Could you check a few things on this model? Use its own coordinates, in mm. A direction names the side the tool comes from. Give positions to 0.01 mm unless a question says otherwise; leave off trailing zeros. Order: outer loops, then holes, each group sorted by start corner. A loop starts at its lowest first (then second) coordinate and runs counter-clockwise, first axis right, second up.
(1) If we mould it in two halves opening along Y, with no side actions, what happens to faces 1 (the flat face through (-15, -9.35, 59)), 2 (the flat face through (42.605, 0.49, 34.51))? For each: released by +Y, released by -Y, zero draft, split by the parting line, or undercut.
(2) Imagine slicing it at B-B, the plane x = 0. Write out the boundary of the cut face in (y, z), then the cut area to 3 significant figures.
(3) Will these pins go through, and if not, where does the flat tip stop? pin 1 (10 mm diameter, centred on x = -3.5, y = 6.5, fed in from -Z); pin 2 (3.5 mm diameter, centred on y = 33, z = 7.5, fed in from +X); pin 3 (4 mm diameter, centred on y = -22, z = 12.5, fed in from +X).
(4) Imagine slicing it at A-A, the plane y = 0. Write out the boundary of the cut face in (x, z), then the cut area to 3 significant figures.
(5) If I drill on probe 1 along Y at (x, z) = (-17.5, 52.6); probe 2 along X at (y, z) = (14.5, 52); probe 3 along Y at (x, z) = (-18, 65), over which ranges is the centre line in solid material (lowest first)?
(6) Imagine slicing it at D-D, the plane x = -17.5. Write out the boundary of the cut face in (y, z), then the cut area to 3 significant figures.
(7) On a 3-axis mill with a long thin cutter (end or side, diameter ignored), from which of +Z, -Z, +X, -X, +Y, -Y can I reach the whole of each face in a straight line? I mean faces 3 (the flat face through (-33, 0, 3)), 4 (the flat face through (21, 7, 55)), 5 (the flat face through (18, 8, 54.7)), 6 (the flat face through (32, 34, 8)). Say none if no direction works.
(8) Imagine slicing it at C-C, the plane z = 17. Write out the boundary of the cut face in (x, y), then the cut area to 3 significant figures.
from build123d import *

# Parameters (mm, degrees)
SCHIZZO1_W                   = 70
SCHIZZO1_H                   = 70
ESTRUSIONE_ESTRUSIONE1_DEPTH = 70
SCHIZZO3_W                   = 64
SCHIZZO3_H                   = 64
TAGLIO_ESTRUSIONE2_DEPTH     = 67
TAGLIO_ESTRUSIONE1_REACH     = 87.732
SCHIZZO2_R                   = 3.65
TAGLIO_ESTRUSIONE3_START     = -70
SCHIZZO4_W                   = 64
SCHIZZO4_H                   = 64
TAGLIO_ESTRUSIONE3_DEPTH     = 70
SPECCHIA2_START              = -70
SPECCHIA2_COPY_1_SKETCH_W    = 64
SPECCHIA2_COPY_1_SKETCH_H    = 64
SPECCHIA2_COPY_1_DEPTH       = 70
ESTRUSIONE_ESTRUSIONE2_DEPTH = 15.3
SCHIZZO6_R                   = 1.5
TAGLIO_ESTRUSIONE4_DEPTH     = 3
SCHIZZO7_W                   = 42
SCHIZZO7_H                   = 14
SCHIZZO7_H_2                 = 11.35
ESTRUSIONE_ESTRUSIONE3_DEPTH = 8
SCHIZZO8_W                   = 15
SCHIZZO8_H                   = 70


with BuildPart() as part:
    # Schizzo1 → Estrusione-Estrusione1 (new body)
    with BuildSketch(Plane.XY):
        Rectangle(SCHIZZO1_W, SCHIZZO1_H)
    extrude(amount=ESTRUSIONE_ESTRUSIONE1_DEPTH)

    # Schizzo3 → Taglio-Estrusione2 (cut)
    with BuildSketch(Plane(origin=(0, 0, 0), x_dir=(-1, 0, 0), z_dir=(0, 0, -1))):
        Rectangle(SCHIZZO3_W, SCHIZZO3_H)
    extrude(amount=-TAGLIO_ESTRUSIONE2_DEPTH, mode=Mode.SUBTRACT)

    # Schizzo2 → Taglio-Estrusione1 (cut, up to next)
    with BuildSketch(Plane.XY.offset(70), mode=Mode.PRIVATE) as taglio_estrusione1_sk1:
        Circle(SCHIZZO2_R)
    taglio_estrusione1_tool1 = extrude(taglio_estrusione1_sk1.sketch, amount=-TAGLIO_ESTRUSIONE1_REACH, mode=Mode.PRIVATE) & part.part
    add(taglio_estrusione1_tool1.solids().sort_by_distance((0, 0, 70))[0], mode=Mode.SUBTRACT)

    # Schizzo4 → Taglio-Estrusione3 (cut)
    with BuildSketch(Plane.XZ.offset(35).offset(TAGLIO_ESTRUSIONE3_START)):
        with Locations((0, 35)):
            Rectangle(SCHIZZO4_W, SCHIZZO4_H)
    taglio_estrusione3 = extrude(amount=TAGLIO_ESTRUSIONE3_DEPTH, mode=Mode.SUBTRACT)

    # Specchia1: Taglio-Estrusione3 across plane
    add(taglio_estrusione3.mirror(Plane(origin=(0, 0, 0), x_dir=(0, 0, 1), z_dir=(-0.7071067811865476, 0.7071067811865475, 0))), mode=Mode.SUBTRACT)

    # Specchia2: Taglio-Estrusione3 across plane
    add(taglio_estrusione3.mirror(Plane(origin=(0, 0, 0), x_dir=(0, 0, 1), z_dir=(-0.7071067811865476, 0.7071067811865475, 0))), mode=Mode.SUBTRACT)

    # Specchia2 copy 1 sketch → Specchia2 copy 1 (cut)
    with BuildSketch(Plane.XZ.offset(35).offset(SPECCHIA2_START)):
        with Locations((0, 35)):
            Rectangle(SPECCHIA2_COPY_1_SKETCH_W, SPECCHIA2_COPY_1_SKETCH_H)
    extrude(amount=SPECCHIA2_COPY_1_DEPTH, mode=Mode.SUBTRACT)

    # Schizzo5 → Estrusione-Estrusione2 (add)
    with BuildSketch(Plane(origin=(0, 0, 67), x_dir=(-1, 0, 0), z_dir=(0, 0, -1))):
        Polygon((-21, 23.65), (21, 23.65), (21, -9.35), (8, -9.35), (8, 4.65), (-8, 4.65), (-8, -9.35), (-21, -9.35), align=None)
    extrude(amount=ESTRUSIONE_ESTRUSIONE2_DEPTH)

    # Schizzo6 → Taglio-Estrusione4 (cut)
    with BuildSketch(Plane(origin=(0, 0, 51.7), x_dir=(-1, 0, 0), z_dir=(0, 0, -1))):
        with Locations((-17.5, 7.5)):
            Circle(SCHIZZO6_R)
        with Locations(Location((17.5, 7.5, 0), (0, 0, 180))):
            Circle(SCHIZZO6_R)
    extrude(amount=-TAGLIO_ESTRUSIONE4_DEPTH, mode=Mode.SUBTRACT)

    # Schizzo7 → Estrusione-Estrusione3 (add)
    with BuildSketch(Plane(origin=(0, 0, 67), x_dir=(-1, 0, 0), z_dir=(0, 0, -1))):
        with Locations((0, -28)):
            Rectangle(SCHIZZO7_W, SCHIZZO7_H)
        Polygon((32, 32), (32, 35), (21, 35), (21, 23.65), (21, -9.35), (21, -21), (21, -35), (32, -35), (32, -32), (35, -32), (35, 32), align=None)
        with Locations((0, 29.325)):
            Rectangle(SCHIZZO7_W, SCHIZZO7_H_2)
        Polygon((-21, 23.65), (-21, 35), (-32, 35), (-32, 32), (-35, 32), (-35, -32), (-32, -32), (-32, -35), (-21, -35), (-21, -21), (-21, -9.35), align=None)
    extrude(amount=ESTRUSIONE_ESTRUSIONE3_DEPTH)

    # Sweep1: sweep along a path in Schizzo9
    with BuildLine(Plane.XZ.offset(35)) as sweep1_path:
        Line((35, 70), (50, 0))
    # Schizzo8 → Sweep1 (sweep)
    with BuildSketch(Plane(origin=(0, 0, 0), x_dir=(-1, 0, 0), z_dir=(0, 0, -1))):
        with Locations((-42.5, 0)):
            Rectangle(SCHIZZO8_W, SCHIZZO8_H)
    sweep1 = sweep(path=sweep1_path.line)

    # Specchia4: Sweep1 across plane
    add(sweep1.mirror(Plane(origin=(0, 0, 0), x_dir=(0, 0, 1), z_dir=(1, 0, 0))))


solid = part.part
Answer block:
1. face 1: undercut
1. face 2: zero draft
2. outline: (-35, 0) - (-32, 0) - (-32, 3) - (-35, 3) - close; (-35, 59) - (-21, 59) - (-21, 67) - (-3.65, 67) - (-3.65, 70) - (-35, 70) - close; (3.65, 67) - (4.65, 67) - (4.65, 51.7) - (23.65, 51.7) - (23.65, 59) - (35, 59) - (35, 70) - (3.65, 70) - close; (32, 0) - (35, 0) - (35, 3) - (32, 3) - close
2. area: 700 mm2
3. pin 1: stops at z = 51.7
3. pin 2: stops at x = 48.77
3. pin 3: stops at x = 47.75
4. outline: (-50, 0) - (-32, 0) - (-32, 3) - (-34.36, 3) - (-22.36, 59) - (-21, 59) - (-21, 51.7) - (-8, 51.7) - (-8, 67) - (-3.65, 67) - (-3.65, 70) - (-35, 70) - close; (3.65, 67) - (8, 67) - (8, 51.7) - (21, 51.7) - (21, 59) - (22.36, 59) - (34.36, 3) - (32, 3) - (32, 0) - (50, 0) - (35, 70) - (3.65, 70) - close
4. area: 2,620 mm2
5. probe 1: y = -9.35 to 6, 9 to 23.65
5. probe 2: x = -38.86 to -23.86, -21 to 21, 23.86 to 38.86
5. probe 3: y = -35 to -21, -9.35 to 35
6. outline: (-35, 0) - (-32, 0) - (-32, 3) - (-35, 3) - close; (-35, 59) - (-21, 59) - (-21, 67) - (-9.35, 67) - (-9.35, 51.7) - (6, 51.7) - (6, 54.7) - (9, 54.7) - (9, 51.7) - (23.65, 51.7) - (23.65, 59) - (35, 59) - (35, 70) - (-35, 70) - close; (32, 0) - (35, 0) - (35, 3) - (32, 3) - close
6. area: 927 mm2
7. face 3: none
7. face 4: -Z, +Y, -Y
7. face 5: -Z
7. face 6: +Y, -Y
8. outline: (-46.36, -35) - (-31.36, -35) - (-31.36, 35) - (-46.36, 35) - close; (31.36, -35) - (46.36, -35) - (46.36, 35) - (31.36, 35) - close
8. area: 2,100 mm2
